Here's how the part is built. I have some questions about the finished solid (model axes, mm). A direction names the side the tool comes from. Round coordinates to 2 decimals unless told otherwise and drop trailing zeros. Loops run counter-clockwise (first coordinate to the right, second up) from the corner with the lowest first, then second, coordinate; pieces in that order, holes last. Notation, with made-up numbers: (-38, 18.25) -> (7, 18.25) arc R26 cw to (7, 34.25) -> close; hole circle Ø7 at (37.5, 0.25). An arc over 180 degrees is marked (long way). Use CSV: the item, a comma, the result in double quotes. Start each with the question number.
from build123d import *

# Parameters (mm, degrees)
SKETCH006_W          = 20
SKETCH006_H          = 40
PAD001_DEPTH         = 40
SKETCH007_R          = 1.55
POCKET005_DEPTH      = 6
SKETCH008_R          = 1.55
POCKET006_DEPTH      = 6
SKETCH009_R          = 1.55
POCKET007_DEPTH      = 8
SKETCH010_R          = 2.55
POCKET008_DEPTH      = 20
SKETCH011_R          = 2.55
POCKET009_DEPTH      = 14
POCKET010_DEPTH      = 5.5
SKETCH016_R          = 1.55
POCKET014_DEPTH      = 53.206
POCKET014_DEPTH_BACK = 53.206
SKETCH017_R          = 3
POCKET015_DEPTH      = 31.206
SKETCH018_R          = 3
POCKET016_DEPTH      = 31.206
FILLET001_R          = 2


with BuildPart() as part:
    # Sketch006 → Pad001 (new body)
    with BuildSketch(Plane.XY):
        with BuildLine():
            Line((-53.205, 0), (-16.535, 63.5143031136))
            Line((-16.535, 63.5143031136), (-33.8555080757, 73.5143031136))
            Line((-33.8555080757, 73.5143031136), (-21.7278633238, 94.52))
            ThreePointArc((-13.0676092859, 99.52), (-18.0676092859, 98.1802540378), (-21.7278633238, 94.52))
            Line((-13.0676092859, 99.52), (13.0676092859, 99.52))
            ThreePointArc((21.7278633238, 94.52), (18.0676092859, 98.1802540378), (13.0676092859, 99.52))
            Line((33.8555080757, 73.5143031136), (21.7278633238, 94.52))
            Line((16.535, 63.5143031136), (33.8555080757, 73.5143031136))
            Line((53.205, 0), (16.535, 63.5143031136))
            Line((53.205, 0), (48.0088475773, -3))
            Line((48.0088475773, -3), (40.9247597743, 9.27))
            ThreePointArc((40.9247597743, 9.27), (39.0946327554, 11.1001270189), (36.5946327554, 11.77))
            Line((-36.5946327554, 11.77), (36.5946327554, 11.77))
            ThreePointArc((-36.5946327554, 11.77), (-39.0946327554, 11.1001270189), (-40.9247597743, 9.27))
            Line((-48.0088475773, -3), (-40.9247597743, 9.27))
            Line((-53.205, 0), (-48.0088475773, -3))
        make_face()
        with Locations((0, 73.52)):
            Rectangle(SKETCH006_W, SKETCH006_H, mode=Mode.SUBTRACT)
        with BuildLine():
            Line((-23.4599141314, 39.52), (-34.2852316787, 20.77))
            ThreePointArc((-34.2852316787, 20.77), (-34.2852316787, 18.77), (-32.5531808711, 17.77))
            Line((-32.5531808711, 17.77), (32.5531808711, 17.77))
            ThreePointArc((32.5531808711, 17.77), (34.2852316787, 18.77), (34.2852316787, 20.77))
            Line((34.2852316787, 20.77), (23.4599141314, 39.52))
            ThreePointArc((23.4599141314, 39.52), (20.5317109011, 42.4482032303), (16.5317109011, 43.52))
            Line((16.5317109011, 43.52), (-16.5317109011, 43.52))
            ThreePointArc((-16.5317109011, 43.52), (-20.5317109011, 42.4482032303), (-23.4599141314, 39.52))
        make_face(mode=Mode.SUBTRACT)
    extrude(amount=PAD001_DEPTH)

    # Sketch007 (on DatumPlane) → Pocket005 (cut, symmetric)
    with BuildSketch(Plane(origin=(53, 0, 0), x_dir=(-0.5, 0.8660254038, 0), z_dir=(0.8660254038, 0.5, 0))):
        with Locations((47.2375, 30)):
            Circle(SKETCH007_R)
        with Locations((9.8975, 30)):
            Circle(SKETCH007_R)
        with Locations((47.2375, 10)):
            Circle(SKETCH007_R)
        with Locations((9.8975, 10)):
            Circle(SKETCH007_R)
    extrude(amount=POCKET005_DEPTH, both=True, mode=Mode.SUBTRACT)

    # Sketch008 (on DatumPlane) → Pocket006 (cut, symmetric)
    with BuildSketch(Plane(origin=(-53, 0, 0), x_dir=(0.5, 0.8660254038, 0), z_dir=(0.8660254038, -0.5, 0))):
        with Locations((47.2375, 30)):
            Circle(SKETCH008_R)
        with Locations((47.2375, 10)):
            Circle(SKETCH008_R)
        with Locations((9.8975, 10)):
            Circle(SKETCH008_R)
        with Locations((9.8975, 30)):
            Circle(SKETCH008_R)
    extrude(amount=POCKET006_DEPTH, both=True, mode=Mode.SUBTRACT)

    # Sketch009 → Pocket007 (cut)
    with BuildSketch(Plane(origin=(0, 99.52, 0), x_dir=(-1, 0, 0), z_dir=(0, 1, 0))):
        with Locations((0, 30)):
            Circle(SKETCH009_R)
        with Locations((0, 10)):
            Circle(SKETCH009_R)
    extrude(amount=-POCKET007_DEPTH, mode=Mode.SUBTRACT)

    # Sketch010 → Pocket008 (cut)
    with BuildSketch(Plane.XZ):
        with Locations((0, 20)):
            Circle(SKETCH010_R)
    extrude(amount=-POCKET008_DEPTH, mode=Mode.SUBTRACT)

    # Sketch011 → Pocket009 (cut)
    with BuildSketch(Plane.XZ.offset(-53.52)):
        with Locations((0, 20)):
            Circle(SKETCH011_R)
    extrude(amount=POCKET009_DEPTH, mode=Mode.SUBTRACT)

    # Sketch012 → Pocket010 (cut)
    with BuildSketch(Plane.XZ.offset(-53.52)):
        Polygon((4.1, 17.6328638963), (4.1, 22.3671361037), (0, 24.7342722074), (-4.1, 22.3671361037), (-4.1, 17.6328638963), (0, 15.2657277926), align=None)
    extrude(amount=POCKET010_DEPTH, mode=Mode.SUBTRACT)

    # Sketch016 → Pocket014 (cut, two sides)
    with BuildSketch(Plane.YZ) as pocket014_sk:
        with Locations((83.52, 30)):
            Circle(SKETCH016_R)
        with Locations((83.52, 10)):
            Circle(SKETCH016_R)
    extrude(amount=-POCKET014_DEPTH, mode=Mode.SUBTRACT)
    extrude(pocket014_sk.sketch, amount=POCKET014_DEPTH_BACK, mode=Mode.SUBTRACT)

    # Sketch017 → Pocket015 (cut, through all)
    with BuildSketch(Plane.YZ.offset(22)):
        with Locations((83.52, 30)):
            Circle(SKETCH017_R)
        with Locations((83.52, 10)):
            Circle(SKETCH017_R)
    extrude(amount=POCKET015_DEPTH, mode=Mode.SUBTRACT)

    # Sketch018 → Pocket016 (cut, through all)
    with BuildSketch(Plane.YZ.offset(-22)):
        with Locations((83.52, 30)):
            Circle(SKETCH018_R)
        with Locations((83.52, 10)):
            Circle(SKETCH018_R)
    extrude(amount=-POCKET016_DEPTH, mode=Mode.SUBTRACT)

    # Fillet001
    fillet001_edges = [part.edges().sort_by_distance(p)[0] for p in [
        (27.791686, 84.017152, 40),
        (18.067609, 98.180254, 40),
        (0, 99.52, 40),
        (-18.067609, 98.180254, 40),
        (-27.791686, 84.017152, 40),
        (27.791686, 84.017152, 0),
        (18.067609, 98.180254, 0),
        (0, 99.52, 0),
        (-18.067609, 98.180254, 0),
        (-27.791686, 84.017152, 0),
    ]]
    fillet(fillet001_edges, radius=FILLET001_R)


solid = part.part
Q1. If we mould it in two halves opening along Z, with no side actions, what happens to faces 5 (the flat face through (0, 51, 0)), 6 (the flat face through (0, 51, 40)), 7 (the cylindrical face through (1.18, 45.8, 17.74))? For each: pulls with the +Z half, pulls with the -Z half, needs draft (parallel to the pull), parting line crosses it, or undercut.
Q2. Will these pins go through, and if not, where does the flat tip stop? pin 1 Ø10 at (x, z) = (33, 32) entering from -Y; pin 2 Ø3.5 at (y, z) = (83.52, 10) entering from +X; pin 3 Ø6.5 at (y, z) = (82.5, 29.5) entering from +X.
Q3. I want a section at C-C, the plane y = 13. List the corners of the cut face in (x, z) for me, then the cut area to 3 significant figures.
Q4. I need wall thicknesses on line 1 along Z through (x, y) = (-13.25, 83.52); line 2 along Y through (x, z) = (1, 25.5); line 3 along Y through (x, z) = (14.5, 10). Which ranges of each line are inside material? Lowest first, please.
Q5. I want a section at A-A, the plane y = 66. List the corners of the cut face in (x, z) for me, then the cut area to 3 significant figures.
Q6. I want a section at B-B, the plane z = 30. Count the separate pieces of the cut face and the enclosed holes in it, then the cut area to 3 significant figures.
Q7. I want a section at D-D, the plane y = 30.5. List the corners of the cut face in (x, z) for me.
Q8. For faces 1 (the flat face through (-2.02, 50.81, 23.57)), 2 (the flat face through (-25.07, 68.44, 19.72)), 3 (the cylindrical face through (0.336, 96.562, 8.487)), 4 (the flat face through (0, 53.52, 15)), which set-ups out of +Z, -Z, +X, -X, +Y, -Y let a thin tool reach every point of the face, with its end or its side?
Values found:
1,face 5,"pulls with the -Z half"
1,face 6,"pulls with the +Z half"
1,face 7,"undercut"
2,pin 1,"y = 11.57"
2,pin 2,"x = 22"
2,pin 3,"x = 30.54"
3,outline,"(-45.7, 0) -> (45.7, 0) -> (45.7, 40) -> (-45.7, 40) -> close; hole circle Ø5.1 at (0, 20)"
3,area,"3,640 mm2"
4,line 1,"0 to 8.45, 11.55 to 28.45, 31.55 to 40"
4,line 2,"11.77 to 17.77, 43.52 to 53.52, 93.52 to 99.52"
4,line 3,"11.77 to 17.77, 43.52 to 81.97, 85.07 to 99.42"
5,outline,"(-20.84, 0) -> (-10, 0) -> (-10, 40) -> (-20.84, 40) -> close; (10, 0) -> (20.84, 0) -> (20.84, 40) -> (10, 40) -> close"
5,area,"867 mm2"
6,separate pieces,"6"
6,enclosed holes,"0"
6,area,"2,810 mm2"
7,outline,"(-35.6, 0) -> (-28.67, 0) -> (-28.67, 40) -> (-35.6, 40) -> close; (28.67, 0) -> (35.6, 0) -> (35.6, 40) -> (28.67, 40) -> close"
8,face 1,"none"
8,face 2,"+Z, -Z, -X"
8,face 3,"+Y"
8,face 4,"+Z, -Z"
